Job drawing, mm, ordinate dimensions from the low corner. One solid piece. Coordinates: 2 decimals unless noted, no trailing zeros. Order: outer loops, then holes, each group sorted by start corner. A loop starts at its lowest first (then second) coordinate and runs counter-clockwise, first axis right, second up. Notation, with made-up numbers: (54, 1.25) - (59, 1.25) arc R14 cw to (59, 8.25) - close; hole circle Ø5 at (71, 10.25). An arc over 180 degrees is marked (long way). Return JSON: item names as keys, results as strings.
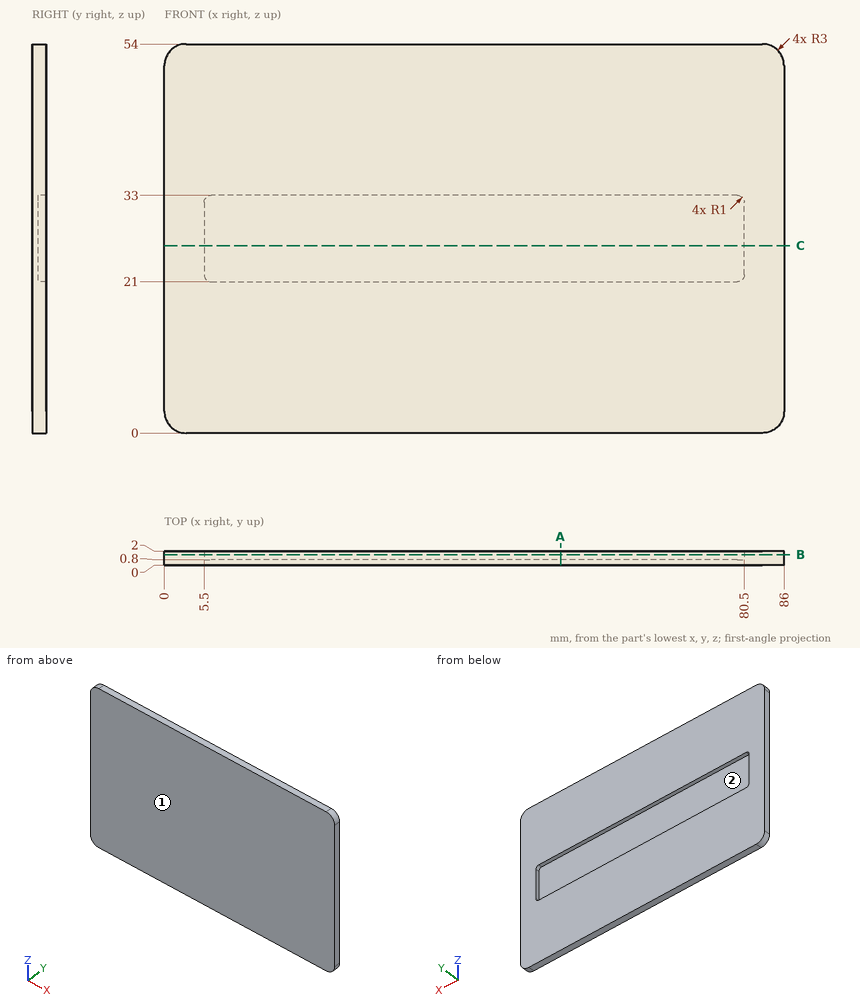
1. Mould opens along X. For the marked faces 1 and 2 say: pulls with the +X half, pulls with the -X half, needs draft (parallel to the pull), parting line crosses it, or undercut.
Check values:
{"face 1": "needs draft", "face 2": "undercut"}
2. Probe L1, parallel to Z at x = 21.5, y = 1.5; L2, parallel to Y at x = 45, z = 26; L3, parallel to X at y = 0.5, z = 2. List the from-to ranges inside material, lowest first.
Check values:
{"L1": "0 to 21, 33 to 54", "L2": "0 to 0.8", "L3": "0.17 to 85.83"}
3. Cut at A-A on x = 55. Give the cut face in (y, z).
Check values:
{"outline": "(0, 0) - (2, 0) - (2, 21) - (0.8, 21) - (0.8, 33) - (2, 33) - (2, 54) - (0, 54) - close"}
4. Cut at B-B on y = 1.5. Give the cut face in (x, z).
Check values:
{"outline": "(0, 3) arc R3 ccw to (3, 0) - (83, 0) arc R3 ccw to (86, 3) - (86, 51) arc R3 ccw to (83, 54) - (3, 54) arc R3 ccw to (0, 51) - close; hole (5.5, 22) arc R1 ccw to (6.5, 21) - (79.5, 21) arc R1 ccw to (80.5, 22) - (80.5, 32) arc R1 ccw to (79.5, 33) - (6.5, 33) arc R1 ccw to (5.5, 32) - close"}
5. Cut at C-C on z = 26. Give the cut face in (x, y).
Check values:
{"outline": "(0, 0) - (86, 0) - (86, 2) - (80.5, 2) - (80.5, 0.8) - (5.5, 0.8) - (5.5, 2) - (0, 2) - close"}
